Answer from the drawing. Dimensions are ordinates in mm from the lowest x, y and z of the part. Coordinates: 2 decimals unless noted, no trailing zeros. Order: outer loops, then holes, each group sorted by start corner. A loop starts at its lowest first (then second) coordinate and runs counter-clockwise, first axis right, second up. Notation, with made-up numbers: (69, 42.25) -> (93, 42.25) arc R29 cw to (93, 76.25) -> close; hole circle Ø6 at (-7, 85). An arc over 180 degrees is marked (long way). Answer in a Markdown table with one row per item.
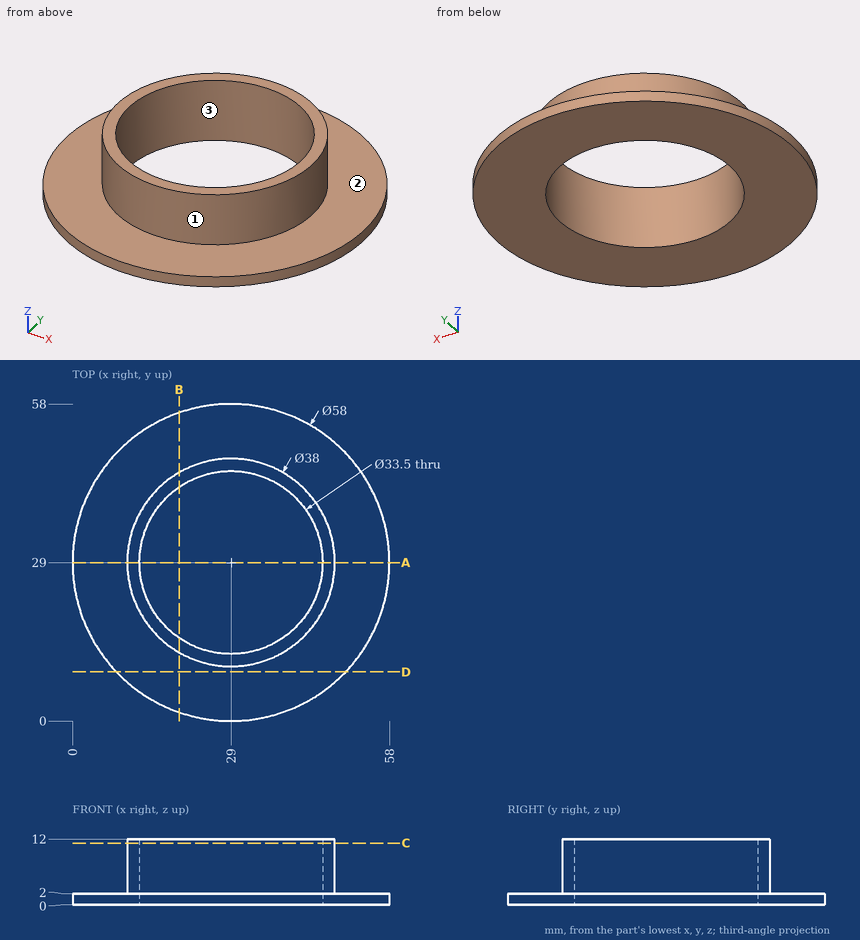
Q1. Given pin 1 (5 mm diameter, centred on x = 9, y = 18, fed in from +Z); pin 2 (10 mm diameter, centred on x = 10, y = 49.5, fed in from -Z); pin 3 (4 mm diameter, centred on y = 18.5, z = 3.5, fed in from +X); pin 4 (1.5 mm diameter, centred on x = 18.5, z = 9, fed in from +Y), each flat-ended and moving along its own axis, determine where each tip first touches the part or whether it passes through.
Outcome:
| item | result |
|---|---|
| pin 1 | z = 2 |
| pin 2 | z = 0 |
| pin 3 | x = 56.51 |
| pin 4 | y = 45.31 |
Q2. The part is cut by section B-B (x = 19.5). Write down the section's boundary in (y, z), then the cut area to 3 significant figures.
Outcome:
| item | result |
|---|---|
| outline | (1.6, 0) -> (15.2, 0) -> (15.2, 12) -> (12.55, 12) -> (12.55, 2) -> (1.6, 2) -> close; (42.8, 0) -> (56.4, 0) -> (56.4, 2) -> (45.45, 2) -> (45.45, 12) -> (42.8, 12) -> close |
| area | 108 mm² |
Q3. The part is cut by section D-D (y = 9). Write down the section's boundary in (x, z).
Outcome:
| item | result |
|---|---|
| outline | (8, 0) -> (50, 0) -> (50, 2) -> (8, 2) -> close |
Q4. The part is cut by section A-A (y = 29). Write down the section's boundary in (x, z).
Outcome:
| item | result |
|---|---|
| outline | (0, 0) -> (12.25, 0) -> (12.25, 12) -> (10, 12) -> (10, 2) -> (0, 2) -> close; (45.75, 0) -> (58, 0) -> (58, 2) -> (48, 2) -> (48, 12) -> (45.75, 12) -> close |
Q5. For a pull along Y with two mould halves and no side action, classify the marked faces 1, 2 and 3 as pulls with the +Y half, pulls with the -Y half, needs draft (parallel to the pull), parting line crosses it, or undercut.
Outcome:
| item | result |
|---|---|
| face 1 | parting line crosses it |
| face 2 | needs draft |
| face 3 | undercut |
Q6. Consider line 1 (Y direction, x = 29, z = 9.5); line 2 (X direction, y = 28.5, z = 3); line 3 (Z direction, x = 10, y = 16.5). Determine where each line is inside the solid, lowest interval first.
Outcome:
| item | result |
|---|---|
| line 1 | 10 to 12.25, 45.75 to 48 |
| line 2 | 10.01 to 12.26, 45.74 to 47.99 |
| line 3 | 0 to 2 |
Q7. The part is cut by section C-C (z = 11.25). Write down the section's boundary in (x, y), then the cut area to 3 significant figures.
Outcome:
| item | result |
|---|---|
| outline | circle Ø38 at (29, 29); hole circle Ø33.5 at (29, 29) |
| area | 253 mm² |
